Verification items for the finished model (mm, model axes). Face numbers are marked on the shaded views. A direction names the side the tool comes from. Round coordinates to 2 decimals unless told otherwise and drop trailing zeros. Write each loop counter-clockwise with the first axis right and the second up, starting at its lowest first coordinate (ties: lowest second). Pieces come first, ordered by that corner, then holes. Notation, with made-up numbers: M 54.5,50.5 L 104.5,50.5 A9 ccw 104.5,57.5 Z; hole C -1.75,68 d3. An arc over 180 degrees is marked long. One line per question, with ' | ' between items.
from build123d import *

# Parameters (mm, degrees)
F0_W     = 38.1
F0_H     = 3.81
F1_DEPTH = 7.62
F2_W     = 13.867821
F2_H     = 3.260234
F3_DEPTH = 19.05
F4_W     = 5.08
F4_H     = 2.54
F5_DEPTH = 6.35
F6_W     = 4.791245
F6_H     = 2.137142
F7_DEPTH = 5.08


with BuildPart() as f1:
    # F0 (on Top) → F1 (new body)
    with BuildSketch(Plane.XY):
        with Locations((-46.713926, 5.953849)):
            Rectangle(F0_W, F0_H)
    extrude(amount=F1_DEPTH)

    # F2 (on face) → F3 (join)
    with BuildSketch(Plane(origin=(0, 7.858849, 0), x_dir=(-1, 0, 0), z_dir=(0, 1, 0))):
        with Locations((40.561947, 3.81)):
            Rectangle(F2_W, F2_H)
    extrude(amount=F3_DEPTH)

    # F4 (on face) → F5 (join)
    with BuildSketch(Plane(origin=(0, 7.858849, 0), x_dir=(-1, 0, 0), z_dir=(0, 1, 0))):
        with Locations((61.318926, 3.81)):
            Rectangle(F4_W, F4_H)
    extrude(amount=F5_DEPTH)

    # F6 (on face) → F7 (join)
    with BuildSketch(Plane.XY.offset(7.62)):
        with Locations((-61.35144, 5.11742)):
            Rectangle(F6_W, F6_H)
    extrude(amount=F7_DEPTH)

    # F8: F1 across face


with BuildPart() as f1_1:
    add(f1.part)
    add(f1.part.mirror(Plane(origin=(-47.846159, 4.048849, 4.301182), x_dir=(1, 0, 0), z_dir=(0, -1, 0))))


solid = f1_1.part
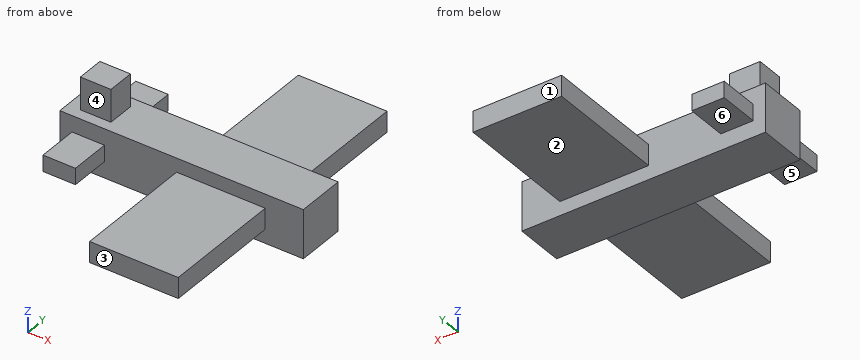
1. Section check B-B, the plane x = -38.5. Record the cut outline in (y, z), then the cut area to 3 significant figures.
Results:
outline: M -18.81,2.18 L 0.24,2.18 L 0.24,0 L 7.86,0 L 7.86,2.18 L 26.91,2.18 L 26.91,5.44 L 7.86,5.44 L 7.86,7.62 L 0.24,7.62 L 0.24,5.44 L -18.81,5.44 Z | area: 182 mm2
2. Tool access check on the marked faces 4, 5 and 6. Record the directions out of +Z, -Z, +X, -X, +Y, -Y that give a thin tool (end or side, any length) a straight path to the whole face; none if there is none.
Results:
face 4: +Z, +X, -X, -Y | face 5: -Z, -X, -Y | face 6: -Z, -X, +Y
3. Section check A-A, the plane y = -4. Record the cut outline in (x, z), then the cut area to 3 significant figures.
Results:
outline: M -63.86,2.54 L -58.78,2.54 L -58.78,5.08 L -63.86,5.08 Z; M -47.5,2.18 L -33.63,2.18 L -33.63,5.44 L -47.5,5.44 Z | area: 58.1 mm2
4. Section check C-C, the plane y = 5.5. Record the cut outline in (x, z).
Results:
outline: M -65.76,0 L -27.66,0 L -27.66,7.62 L -58.96,7.62 L -58.96,12.7 L -63.75,12.7 L -63.75,7.62 L -65.76,7.62 Z
5. Go/stop test with flat-tipped pins: P1, Ø6, axis at x = -51.5, z = 8, coming from the +Y side; P2, Ø11, axis at x = -42, y = 18.5, coming from the -Z side; P3, Ø1.6, axis at y = 17, z = 4, coming from the -X side; P4, Ø1.5, axis at x = -49, y = -4, coming from the -Z side. Record where each tip stops, or that it passes through.
Results:
P1: stops at y = 7.86 | P2: stops at z = 2.18 | P3: stops at x = -47.5 | P4: passes through
6. Section check D-D, the plane z = 11.75. Record the cut outline in (x, y).
Results:
outline: M -63.75,1.91 L -58.96,1.91 L -58.96,6.19 L -63.75,6.19 Z
7. Mould release check, pull along Y, two halves, no side actions. Record for the marked faces 1, 2 and 3: pulls with the +Y half, pulls with the -Y half, needs draft (parallel to the pull), parting line crosses it, or undercut.
Results:
face 1: pulls with the +Y half | face 2: needs draft | face 3: pulls with the -Y half
8. Thickness scan on line 1 (Z direction, x = -45, y = -13); line 2 (Y direction, x = -56, z = 4.25); line 3 (X direction, y = 2, z = 10). Record the ranges inside material, lowest first.
Results:
line 1: z = 2.18 to 5.44 | line 2: y = 0.24 to 7.86 | line 3: x = -63.75 to -58.96
